Input: part model. Units: mm. Frame: model coordinates. Face numbers are marked on the shaded views. A direction names the side the tool comes from. Round coordinates to 2 decimals unless told otherwise and drop trailing zeros. Order: outer loops, then holes, each group sorted by start corner. A loop starts at its lowest first (then second) coordinate and runs counter-clockwise, first axis right, second up. Notation, with made-up numbers: (-17, -37) -> (38, -37) arc R10 cw to (38, -21) -> close; hole circle Ø2 at (-26.5, -15.5). An arc over 180 degrees is marked (long way). Use a Markdown table: item, result.
from build123d import *

# Parameters (mm, degrees)
SKETCH_1_W                = 47
SKETCH_1_H                = 18
EXTRUDE_1_DEPTH           = 6
EXTRUDE_2_DEPTH           = 8
EXTRUDE_2_DEPTH_BACK      = 6
SKETCH_15_W               = 49
SKETCH_15_H               = 22
EXTRUDE_3_DEPTH           = 5
SKETCH_12_W               = 2
SKETCH_12_H               = 8
CUT_EXTRUDE_5_DEPTH       = 37
SKETCH_19_W               = 10
SKETCH_19_H               = 8
EXTRUDE_4_DEPTH           = 3
SKETCH_13_R               = 1
CUT_EXTRUDE_6_DEPTH       = 8
CUT_EXTRUDE_START         = -2.844
SKETCH_5_W                = 25
SKETCH_5_H                = 25
CUT_EXTRUDE_1_DEPTH       = 2.844
HOLE_WIZARD_2_D           = 4.5
HOLE_WIZARD_2_CBORE_D     = 8
HOLE_WIZARD_2_CBORE_DEPTH = 4.6
HOLE_WIZARD_M4_4_D        = 3.3
SKETCH_17_W               = 20.485510756
SKETCH_17_H               = 2.844
CUT_EXTRUDE_8_DEPTH       = 0.5
SKETCH_18_R               = 1
CUT_EXTRUDE_9_DEPTH       = 2.844
FILLET_1_R                = 1


with BuildPart() as part:
    # 草图1 → 凸台-拉伸1 (new body)
    with BuildSketch(Plane(origin=(0, 0, 0), x_dir=(1, 0, 0), z_dir=(0, 1, 0))):
        Rectangle(SKETCH_1_W, SKETCH_1_H)
    extrude(amount=EXTRUDE_1_DEPTH)

    # 草图2 → 凸台-拉伸2 (add, two sides: drawn at the far end of the back side and taken through both)
    with BuildSketch(Plane(origin=(0, 6, 0), x_dir=(1, 0, 0), z_dir=(0, 1, 0)).offset(-EXTRUDE_2_DEPTH_BACK)):
        Polygon((23.5, 9), (-23.5, 9), (-23.5, 11), (25.5, 11), (25.5, -11), (-23.5, -11), (-23.5, -9), (23.5, -9), align=None)
    extrude(amount=EXTRUDE_2_DEPTH + EXTRUDE_2_DEPTH_BACK)

    # 草图15 → 凸台-拉伸3 (add)
    with BuildSketch(Plane(origin=(0, 0, 10), x_dir=(1, 0, 0), z_dir=(0, 1, 0))):
        with Locations((1, 10)):
            Rectangle(SKETCH_15_W, SKETCH_15_H)
    extrude(amount=-EXTRUDE_3_DEPTH)

    # 草图12 → 切除-拉伸5 (cut)
    with BuildSketch(Plane.ZY.offset(23.5)):
        with Locations((10, 10)):
            Rectangle(SKETCH_12_W, SKETCH_12_H)
    extrude(amount=-CUT_EXTRUDE_5_DEPTH, mode=Mode.SUBTRACT)

    # 草图19 → 凸台-拉伸4 (add)
    with BuildSketch(Plane(origin=(0, 0, 9), x_dir=(-1, 0, 0), z_dir=(0, 0, -1))):
        with Locations((-18.5, 10)):
            Rectangle(SKETCH_19_W, SKETCH_19_H)
    extrude(amount=EXTRUDE_4_DEPTH)

    # 草图13 → 切除-拉伸6 (cut)
    with BuildSketch(Plane(origin=(0, 14, 0), x_dir=(1, 0, 0), z_dir=(0, 1, 0))):
        with Locations((23.5, 9)):
            Circle(SKETCH_13_R)
    extrude(amount=-CUT_EXTRUDE_6_DEPTH, mode=Mode.SUBTRACT)

    # 草图5 → 切除-拉伸1 (cut)
    with BuildSketch(Plane.XZ.offset(5).offset(CUT_EXTRUDE_START)):
        with Locations((5.878, -3.014489244)):
            Rectangle(SKETCH_5_W, SKETCH_5_H)
    extrude(amount=CUT_EXTRUDE_1_DEPTH, mode=Mode.SUBTRACT)

    # 打孔尺寸(%根据)内六角圆柱头螺钉的类型2 (through all)
    with Locations(Plane(origin=(-0.122, -5, -0.014489244), x_dir=(0, 0, -1), z_dir=(0, -1, 0))):
        with Locations((0, 0)):
            CounterBoreHole(HOLE_WIZARD_2_D / 2, HOLE_WIZARD_2_CBORE_D / 2, HOLE_WIZARD_2_CBORE_DEPTH)

    # M4 螺纹孔4 (through all)
    with Locations(Plane(origin=(5.878, -2.156, -3.014489244), x_dir=(0, 0, -1), z_dir=(0, -1, 0))):
        with Locations((0, 0)):
            Hole(HOLE_WIZARD_M4_4_D / 2)

    # 草图17 → 切除-拉伸8 (cut)
    with BuildSketch(Plane.ZY.offset(-18.378)):
        with Locations((-0.757244622, -3.578)):
            Rectangle(SKETCH_17_W, SKETCH_17_H)
    extrude(amount=-CUT_EXTRUDE_8_DEPTH, mode=Mode.SUBTRACT)

    # 草图18 → 切除-拉伸9 (cut)
    with BuildSketch(Plane(origin=(0, -5, 0), x_dir=(-1, 0, 0), z_dir=(0, -1, 0))):
        with Locations((6.622, -9.485510756)):
            Circle(SKETCH_18_R)
    extrude(amount=-CUT_EXTRUDE_9_DEPTH, mode=Mode.SUBTRACT)

    # 圆角1
    fillet_1_edges = [part.edges().sort_by_distance(p)[0] for p in [
        (18.878, -3.578, 9.485510756),
    ]]
    fillet(fillet_1_edges, radius=FILLET_1_R)


solid = part.part
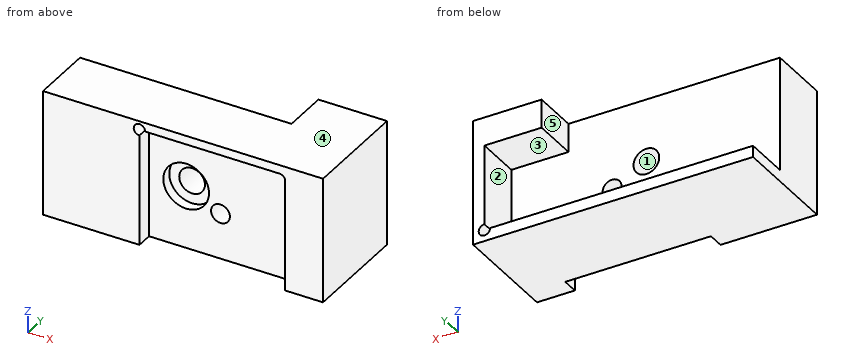
1) Cut plane A-A on y = 11.25. Return loops of the section in (x, z).
Results found:
| item | result |
|---|---|
| outline | (-23.5, -11) -> (25.5, -11) -> (25.5, 11) -> (13.5, 11) -> (13.5, 6) -> (23.5, 6) -> (23.5, -8) arc R1 cw (long way) to (22.5, -9) -> (-23.5, -9) -> close |
2) Cut plane D-D on y = -1.25. Return loops of the section in (x, z), and give its area (3 significant figures).
Results found:
| item | result |
|---|---|
| outline | (-23.5, -11) -> (25.5, -11) -> (25.5, 11) -> (-23.5, 11) -> close; hole circle Ø8 at (-0.12, -0.01); hole circle Ø3.3 at (5.88, -3.01) |
| area | 1,020 mm² |
3) Set-up query: the marked faces 1 and 2. Return all of +Z, -Z, +X, -X, +Y, -Y with unobstructed straight access to the full face (end or side cutting, diameter ignored); none if empty.
Results found:
| item | result |
|---|---|
| face 1 | +Y, -Y |
| face 2 | -X, +Y |
4) Pull-direction query (Z, two-part tool) for the marked faces 3, 4 and 5; classes: +Z half, -Z half, draft (parallel to the pull), parting line (faces both ways), or undercut.
Results found:
| item | result |
|---|---|
| face 3 | undercut |
| face 4 | +Z half |
| face 5 | draft |
5) Cut plane C-C on z = 3. Return loops of the section in (x, y).
Results found:
| item | result |
|---|---|
| outline | (-23.5, -5) -> (-6.62, -5) -> (-6.62, -2.16) -> (-2.75, -2.16) -> (-2.75, -0.4) -> (2.51, -0.4) -> (2.51, -2.16) -> (18.88, -2.16) -> (18.88, -5) -> (25.5, -5) -> (25.5, 14) -> (23.5, 14) -> (23.5, 6) -> (-23.5, 6) -> close |
6) Line query: L1, parallel to Y at x = 4, z = 4; L2, parallel to Z at x = 21, y = 11.5; L3, parallel to Y at x = -12, z = -1.5. Output: solid intervals per line, ascending. Write a range as [from, to].
Results found:
| item | result |
|---|---|
| L1 | y = [-2.16, 6] |
| L2 | z = [-11, -9], [6, 11] |
| L3 | y = [-5, 6] |
7) Pin query (flat end, axial travel): pin 1 Ø2.5 at (x, z) = (-6.62, 9.49) entering from +Y; pin 2 Ø5.5 at (y, z) = (12, 8) entering from -X; pin 3 Ø5 at (x, z) = (-0.12, -0.01) entering from -Y. Return the tip coordinate at first contact, or that it passes through.
Results found:
| item | result |
|---|---|
| pin 1 | stops at y = 6 |
| pin 2 | stops at x = 13.5 |
| pin 3 | stops at y = -0.4 |
8) Cut plane B-B on x = 9. Return loops of the section in (y, z), and give its area (3 significant figures).
Results found:
| item | result |
|---|---|
| outline | (-5, 9.49) -> (-2.16, 9.49) -> (-2.16, -11) -> (14, -11) -> (14, -9) -> (6, -9) -> (6, 11) -> (-5, 11) -> close |
| area | 200 mm² |
